Here's how the part is built. I have some questions about the finished solid (model axes, mm). Face numbers are marked on the shaded views. A direction names the side the tool comes from. Give positions to 0.01 mm unless a question says otherwise; leave off trailing zeros. Loops run counter-clockwise (first coordinate to the right, second up) from the corner with the lowest first, then second, coordinate; pieces in that order, holes last.
Q1. Will these pins go through, and if not, where does the flat tip stop? P1, Ø10, axis at x = 1473, z = 1503.5, coming from the +Y side; P2, Ø4.5, axis at y = -326, z = 1510, coming from the -X side; P3, Ø12, axis at y = -304.5, z = 1512, coming from the -X side.
Q2. If we section it at A-A (z = 1510): Please give me the cut outline in (x, y), plus the area to 3 significant figures.
Q3. If we section it at C-C (y = -294): Please give me the cut outline in (x, z), plus the area to 3 significant figures.
Q4. For the marked faces 1 and 2, which set-ups out of +Z, -Z, +X, -X, +Y, -Y let a thin tool reach every point of the face, with its end or its side?
Q5. If we section it at B-B (y = -347.5): Please give me the cut outline in (x, z), plus the area to 3 significant figures.
Q6. I need wall thicknesses on line 1 (Z direction, x = 1486, y = -294); line 2 (Y direction, x = 1484, z = 1510); line 3 (X direction, y = -331.5, z = 1493.5). Which ranges of each line are inside material? Lowest first, please.
Q7. If we section it at D-D (x = 1476.5): Please give me the cut outline in (y, z).
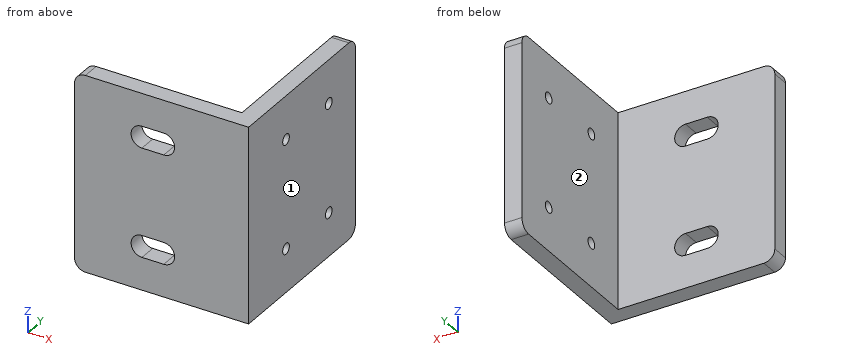
from build123d import *

# Parameters (mm, degrees)
PAD001_DEPTH            = 45
SKETCH_R                = 2.5
POCKET_DEPTH            = 8.001
POCKET001_DEPTH         = 8.001
FILLET001_R             = 5
BODY001_PLACEMENT_ANGLE = 90


with BuildPart() as part:
    # Sketch003 → Pad001 (new body, symmetric)
    with BuildSketch(Plane.XY):
        Polygon((0, 0), (0, 80), (8, 80), (8, 8), (80, 8), (80, 0), align=None)
    extrude(amount=PAD001_DEPTH, both=True)

    # Sketch (on Face4 of Pad001) → Pocket (cut, through all)
    with BuildSketch(Plane(origin=(0, 8, 0), x_dir=(-1, 0, 0), z_dir=(0, 1, 0))):
        with Locations((-60, 25)):
            Circle(SKETCH_R)
        with Locations((-28, -25)):
            Circle(SKETCH_R)
        with Locations((-28, 25)):
            Circle(SKETCH_R)
        with Locations((-60, -25)):
            Circle(SKETCH_R)
    extrude(amount=-POCKET_DEPTH, mode=Mode.SUBTRACT)

    # Sketch007 (on Face11 of Pocket) → Pocket001 (cut, through all)
    with BuildSketch(Plane.YZ.offset(8)):
        with BuildLine():
            ThreePointArc((39, 30), (34, 25), (39, 20))
            Line((39, 20), (49, 20))
            ThreePointArc((49, 20), (54, 25), (49, 30))
            Line((39, 30), (49, 30))
        make_face()
        with BuildLine():
            ThreePointArc((39, -20), (34, -25), (39, -30))
            Line((39, -30), (49, -30))
            ThreePointArc((49, -30), (54, -25), (49, -20))
            Line((39, -20), (49, -20))
        make_face()
    extrude(amount=-POCKET001_DEPTH, mode=Mode.SUBTRACT)

    # Fillet001
    fillet001_edges = [part.edges().sort_by_distance(p)[0] for p in [
        (4, 80, 45),
        (80, 4, 45),
        (4, 80, -45),
        (80, 4, -45),
    ]]
    fillet(fillet001_edges, radius=FILLET001_R)


with BuildPart() as part_1:
    # Body001 placement: moved
    add(part.part.moved(Location((1490, -354, 1485))).rotate(Axis((1490, -354, 1485), (0, 0, 1)), BODY001_PLACEMENT_ANGLE))


solid = part_1.part
Check sheet entries:
1. P1: stops at y = -346
1. P2: passes through
1. P3: stops at x = 1482
2. outline: (1410, -354) - (1436, -354) - (1436, -346) - (1410, -346) - close; (1456, -354) - (1490, -354) - (1490, -328.5) - (1482, -328.5) - (1482, -346) - (1456, -346) - close; (1482, -323.5) - (1490, -323.5) - (1490, -296.5) - (1482, -296.5) - close; (1482, -291.5) - (1490, -291.5) - (1490, -274) - (1482, -274) - close
2. area: 976 mm2
3. outline: (1482, 1440) - (1490, 1440) - (1490, 1457.5) - (1482, 1457.5) - close; (1482, 1462.5) - (1490, 1462.5) - (1490, 1507.5) - (1482, 1507.5) - close; (1482, 1512.5) - (1490, 1512.5) - (1490, 1530) - (1482, 1530) - close
3. area: 640 mm2
4. face 1: +Z, -Z, +X, +Y, -Y
4. face 2: +Z, -Z, -X, +Y
5. outline: (1410, 1445) arc R5 ccw to (1415, 1440) - (1490, 1440) - (1490, 1530) - (1415, 1530) arc R5 ccw to (1410, 1525) - close; hole (1441, 1455) - (1451, 1455) arc R5 ccw to (1451, 1465) - (1441, 1465) arc R5 ccw to start; hole (1441, 1505) - (1451, 1505) arc R5 ccw to (1451, 1515) - (1441, 1515) arc R5 ccw to start
5. area: 6,830 mm2
6. line 1: z = 1440 to 1457.5, 1462.5 to 1507.5, 1512.5 to 1530
6. line 2: y = -354 to -328.5, -323.5 to -296.5, -291.5 to -274
6. line 3: x = 1482 to 1490
7. outline: (-354, 1440) - (-346, 1440) - (-346, 1530) - (-354, 1530) - close
